CAD build for the part. Positions are in the model's coordinates, mm. A direction names the side the tool comes from. Coordinates: 2 decimals unless noted, no trailing zeros. Loops run counter-clockwise (first coordinate to the right, second up) from the corner with the lowest first, then second, coordinate; pieces in that order, holes last. Notation, with made-up numbers: (-10, -21.5) - (19, -21.5) arc R16 ccw to (19, 8.5) - close; hole circle Ø5 at (-24, 53.25). An arc over 180 degrees is marked (long way). Put each result on its own line as item: value.
```python
from build123d import *

# Parameters (mm, degrees)
F1_DEPTH = 3.175
F2_W     = 3.8559212309
F2_H     = 8.382
F3_DEPTH = 12.7
F4_W     = 5.08
F4_H     = 4.445
F5_DEPTH = 129.2387778288
F6_R     = 1.27
F7_DEPTH = 33.402
F8_R     = 1.27
F9_DEPTH = 34.2152275192
F10_R    = 0.762
F11_R    = 0.762


with BuildPart() as f1:
    # F0 (on Front) → F1 (new body)
    with BuildSketch(Plane.XZ):
        with BuildLine():
            ThreePointArc((-18.1050305715, -3.3733308155), (-17.9584921143, -1.6894938048), (-17.9095913851, 0))
            ThreePointArc((-17.9095913851, 0), (-47.1195913851, 29.21), (-76.3295913851, 0))
            Line((-76.3295913851, 0), (-72.5195913851, 0))
            ThreePointArc((-72.5195913851, 0), (-47.1195913851, 25.4), (-21.7195913851, 0))
            ThreePointArc((-21.7195913851, 0), (-45.5289694065, -25.3501463846), (-72.320372623, -3.175))
            Line((-72.320372623, -3.175), (-76.1565243327, -3.175))
            ThreePointArc((-76.1565243327, -3.175), (-47.2193857045, -29.2098295287), (-18.1050305715, -3.3733308155))
        make_face()
        with BuildLine():
            ThreePointArc((-5.2095913851, 0), (-11.5595913851, 3.5657379151), (-17.9095913851, 0))
            ThreePointArc((-17.9095913851, 0), (-17.9584921143, -1.6894938048), (-18.1050305715, -3.3733308155))
            ThreePointArc((-18.1050305715, -3.3733308155), (-11.412472054, -0.5582261258), (-4.9519179152, -3.871290288))
            ThreePointArc((-4.9519179152, -3.871290288), (-5.1451018279, -1.9399280986), (-5.2095913851, 0))
        make_face()
        with BuildLine():
            Line((-72.5195913851, 0), (-76.3295913851, 0))
            ThreePointArc((-76.3295913851, 0), (-76.2862925304, -1.589856692), (-76.1565243327, -3.175))
            Line((-76.1565243327, -3.175), (-72.320372623, -3.175))
            ThreePointArc((-72.320372623, -3.175), (-72.4697377697, -1.5906219786), (-72.5195913851, 0))
        make_face()
        with BuildLine():
            ThreePointArc((53.2104086149, 0), (24.0004086149, 29.21), (-5.2095913851, 0))
            ThreePointArc((-5.2095913851, 0), (-5.1451018279, -1.9399280986), (-4.9519179152, -3.871290288))
            ThreePointArc((-4.9519179152, -3.871290288), (24.3511144785, -29.2078945732), (53.0373415624, -3.175))
            Line((53.0373415624, -3.175), (49.2011898528, -3.175))
            ThreePointArc((49.2011898528, -3.175), (-1.3497377697, 1.5906219786), (49.4004086149, 0))
            Line((49.4004086149, 0), (53.2104086149, 0))
        make_face()
        with BuildLine():
            ThreePointArc((53.0373415624, -3.175), (53.1671097602, -1.589856692), (53.2104086149, 0))
            Line((53.2104086149, 0), (49.4004086149, 0))
            ThreePointArc((49.4004086149, 0), (49.3505549995, -1.5906219786), (49.2011898528, -3.175))
            Line((49.2011898528, -3.175), (53.0373415624, -3.175))
        make_face()
    extrude(amount=F1_DEPTH)

    # F2 (on face) → F3 (join)
    with BuildSketch(Plane.XZ.offset(3.175)):
        with Locations((50.9802258282, 0)):
            Rectangle(F2_W, F2_H)
        Polygon((-75.8977394655, 5.0042275192), (-76.1340230485, -3.3744414722), (-72.2945916673, -3.3733308155), (-72.0217540811, 5.0042275192), align=None)
    extrude(amount=-F3_DEPTH)

    # F4 (on face) → F5 (cut, through all)
    with BuildSketch(Plane.YZ.offset(52.9081864437)):
        with Locations((6.985, 0.4219774121)):
            Rectangle(F4_W, F4_H)
    extrude(amount=-F5_DEPTH, mode=Mode.SUBTRACT)

    # F6 (on face) → F7 (cut, through all)
    with BuildSketch(Plane.XY.offset(4.191)):
        with Locations((51.0031864437, 7.4931297261)):
            Circle(F6_R)
    extrude(amount=-F7_DEPTH, mode=Mode.SUBTRACT)

    # F8 (on face) → F9 (cut, through all)
    with BuildSketch(Plane.XY.offset(5.0042275192)):
        with Locations((-73.9267540811, 7.4932678616)):
            Circle(F8_R)
    extrude(amount=-F9_DEPTH, mode=Mode.SUBTRACT)

    # F10
    f10_edges = [f1.edges().sort_by_distance(p)[0] for p in [
        (49.052265, 9.525, 3.417739),
        (52.908186, 9.525, 3.417739),
        (52.908186, 9.525, -2.995761),
        (49.052265, 9.525, -2.995761),
    ]]
    fillet(f10_edges, radius=F10_R)

    # F11
    f11_edges = [f1.edges().sort_by_distance(p)[0] for p in [
        (-76.11183, 9.525, -2.587482),
        (-75.931013, 9.525, 3.824352),
        (-72.06018, 9.525, 3.824352),
        (-72.26898, 9.525, -2.586927),
    ]]
    fillet(f11_edges, radius=F11_R)


solid = f1.part
```
Q1. Slice it at B-B, the plane x = 42. Give the cut face in (y, z) (3 decimals).
Determined:
outline: (-3.175, -23.005) - (0, -23.005) - (0, -17.921) - (-3.175, -17.921) - close; (-3.175, 17.921) - (0, 17.921) - (0, 23.005) - (-3.175, 23.005) - close
Q2. Slice it at C-C, the plane z = -5.5. Give the cut face in (x, y) (3 decimals).
Determined:
outline: (-75.807, -3.175) - (-71.917, -3.175) - (-71.917, 0) - (-75.807, 0) - close; (-22.322, -3.175) - (-18.432, -3.175) - (-18.432, 0) - (-22.322, 0) - close; (-4.687, -3.175) - (-0.797, -3.175) - (-0.797, 0) - (-4.687, 0) - close; (48.798, -3.175) - (52.688, -3.175) - (52.688, 0) - (48.798, 0) - close
Q3. Slice it at A-A, the plane z = -13. Give the cut face in (x, y) (1 decimal), then the cut area to 3 significant figures.
Determined:
outline: (-73.3, -3.2) - (-68.9, -3.2) - (-68.9, 0) - (-73.3, 0) - close; (-25.3, -3.2) - (-21, -3.2) - (-21, 0) - (-25.3, 0) - close; (-2.2, -3.2) - (2.2, -3.2) - (2.2, 0) - (-2.2, 0) - close; (45.8, -3.2) - (50.2, -3.2) - (50.2, 0) - (45.8, 0) - close
area: 55.1 mm2
Q4. Pin check, flat tips, straight feed: pin 1 Ø3 at (x, y) = (51, 7) entering from -Z; pin 2 Ø3 at (x, z) = (50, 1) entering from +Y (3 decimals); pin 3 Ø1 at (y, z) = (-1.5, 1.5) entering from -X; pin 4 Ø1.5 at (y, z) = (2, 18.5) entering from +X. Stop position of each tip, or through.
Determined:
pin 1: z = -4.19
pin 2: y = 4.445
pin 3: x = -76.31
pin 4: through
Q5. Slice it at D-D, the plane x = -67.5. Give the cut face in (y, z) (3 decimals), then the cut area to 3 significant figures.
Determined:
outline: (-3.175, -20.925) - (0, -20.925) - (0, -15.159) - (-3.175, -15.159) - close; (-3.175, 15.159) - (0, 15.159) - (0, 20.925) - (-3.175, 20.925) - close
area: 36.6 mm2
Q6. Wall check: L1, parallel to X at y = -2.5, z = 23; L2, parallel to X at y = -0.75, z = 3; L3, parallel to X at y = 1, z = 0.5. Give the ranges that are in metal, low to high. Write a range as from..to.
Determined:
L1: -65.13..-57.9, -36.34..-29.11, 5.99..13.22, 34.78..42.01
L2: -76.18..-72.09, -21.9..-18.06, -14.4..-8.71, -5.06..-1.22, 49.05..53.06
L3: -76.02..-72.17, 49.05..52.91
Q7. Tool access for faces 1 (the flat face through (-75, 6, -1.801)), 2 (the cylindrical face through (-72.715, 7.875, -2.577)), 3 (the flat face through (-74, 5, 5.004)), 4 (the flat face through (-74, 9.525, 4)), 5 (the flat face through (49.052, 1, 0)): list every direction of +Z, -Z, +X, -X, +Y, -Y with a clear straight run to the whole face (end or side of a thin tool).
Determined:
face 1: +X, -X, +Y
face 2: +Z, -Z
face 3: +Z, +X, -X, +Y
face 4: +Z, -Z, +X, -X, +Y
face 5: +Y, -Y
Q8. Mould opens along Z. For faces 6 (the flat face through (51, 5, 4.191)), 7 (the flat face through (51, 6, -1.801)), 8 (the flat face through (52.908, 3, 0)) say: +Z half, -Z half, draft (parallel to the pull), parting line (faces both ways), or undercut.
Determined:
face 6: +Z half
face 7: undercut
face 8: draft
